Source: CAD feature listing. Evaluate the final solid. Frame: model axes, mm. Face numbers are marked on the shaded views. A direction names the side the tool comes from. Round coordinates to 2 decimals unless told otherwise and drop trailing zeros. Order: outer loops, then holes, each group sorted by start corner. A loop starts at its lowest first (then second) coordinate and runs counter-clockwise, first axis right, second up. Notation, with made-up numbers: M 86,77.25 L 142,77.25 A34 ccw 142,110.25 Z; hole C -36.75,15.5 d1. An arc over 180 degrees is marked long. Answer as CSV lines item,"result". Start each with the question number.
Item 1: Section query B-B on x = 51. Return the cut outline in (y, z).
Item 2: Section query C-C on z = -55. Return the cut outline in (x, y), plus the area to 3 significant figures.
Item 3: Section query D-D on y = 27. Return the cut outline in (x, z), plus the area to 3 significant figures.
Item 4: Set-up query: the marked faces 1 and 2. Return all of +Z, -Z, +X, -X, +Y, -Y with unobstructed straight access to the full face (end or side cutting, diameter ignored); none if empty.
Item 5: Section query A-A on y = 47. Return the cut outline in (x, z), plus the area to 3 significant figures.
Item 6: First-contact query: P1, Ø2, axis at y = 32, z = -28, coming from the +X side; P2, Ø12, axis at x = 28.5, z = -23, coming from the +Y side; P3, Ø1.5, axis at y = 7, z = 2.5, coming from the +X side. Flat tips, straight axial feed; report the tip coordinate or a pass-through.
Item 7: Line query: line 1 (Y direction, x = 24, z = -10); line 2 (X direction, y = 7, z = -67). Output: solid intervals per line, ascending. Write a range as [from, to].
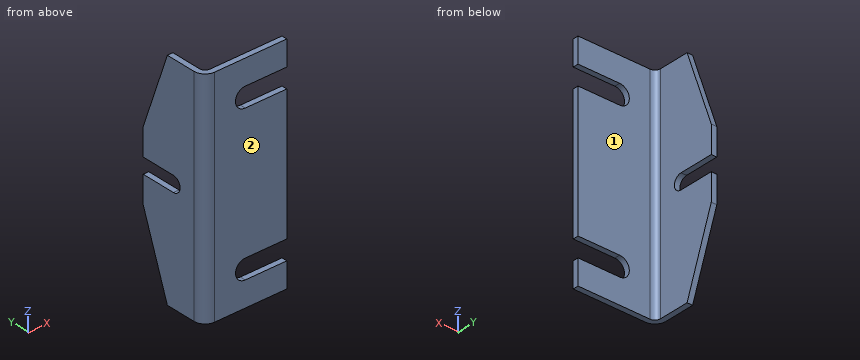
from build123d import *

# Parameters (mm, degrees)
BASE_FLANGE3_DEPTH = 80
CUT_EXTRUDE1_DEPTH = 110.708705215
CUT_EXTRUDE2_DEPTH = 111.072703247


# Sheet-metal steps are written as plain solids
with BuildPart() as part:
    # Sketch1 → Base-Flange3 (new, symmetric)
    with BuildSketch(Plane.XY):
        with BuildLine():
            Line((60, 0), (8, 0))
            ThreePointArc((8, 0), (2.343145751, 2.343145751), (0, 8))
            Line((0, 8), (0, 50))
            Line((0, 50), (4, 50))
            Line((4, 50), (4, 8))
            ThreePointArc((4, 8), (5.171572875, 5.171572875), (8, 4))
            Line((8, 4), (60, 4))
            Line((60, 4), (60, 0))
        make_face()
    extrude(amount=BASE_FLANGE3_DEPTH, both=True)

    # Sketch14 → Cut-Extrude1 (cut, through all)
    with BuildSketch(Plane(origin=(4, 0, 0), x_dir=(0, 0, -1), z_dir=(1, 0, 0))):
        Polygon((-80, 30), (-25, 50), (-80, 50), align=None)
        Polygon((80, 30), (25, 50), (80, 50), align=None)
        with BuildLine():
            Line((-5.5, 50), (-5.5, 25))
            ThreePointArc((-5.5, 25), (0, 19.5), (5.5, 25))
            Line((5.5, 25), (5.5, 50))
            Line((5.5, 50), (-5.5, 50))
        make_face()
    extrude(amount=-CUT_EXTRUDE1_DEPTH, mode=Mode.SUBTRACT)

    # Sketch16 → Cut-Extrude2 (cut, through all)
    with BuildSketch(Plane(origin=(0, 4, 0), x_dir=(1, 0, 0), z_dir=(0, 1, 0))):
        with BuildLine():
            Line((60, 62), (30, 62))
            ThreePointArc((30, 62), (23, 55), (30, 48))
            Line((30, 48), (60, 48))
            Line((60, 48), (60, 62))
        make_face()
        with BuildLine():
            Line((60, -48), (60, -62))
            Line((60, -62), (30, -62))
            ThreePointArc((30, -62), (23, -55), (30, -48))
            Line((30, -48), (60, -48))
        make_face()
    extrude(amount=-CUT_EXTRUDE2_DEPTH, mode=Mode.SUBTRACT)


solid = part.part
Results:
1,outline,"M 0,-80 L 4,-80 L 4,-62 L 0,-62 Z; M 0,-48 L 4,-48 L 4,48 L 0,48 Z; M 0,62 L 4,62 L 4,80 L 0,80 Z"
2,outline,"M 0,8 A8 ccw 8,0 L 23,0 L 23,4 L 8,4 A4 cw 4,8 L 4,39.09 L 0,39.09 Z"
2,area,"222 mm^2"
3,outline,"M 0,-80 L 4,-80 L 4,-5.5 L 0,-5.5 Z; M 0,5.5 L 4,5.5 L 4,80 L 0,80 Z"
3,area,"596 mm^2"
4,face 1,"+Z, -Z, +X, +Y"
4,face 2,"+Z, -Z, +X, -X, -Y"
5,outline,"M 0,-33.25 L 4,-33.25 L 4,-5.5 L 0,-5.5 Z; M 0,5.5 L 4,5.5 L 4,33.25 L 0,33.25 Z"
5,area,"222 mm^2"
6,P1,"x = 4"
6,P2,"y = 4"
6,P3,"x = 4.4"
7,line 1,"[0, 4]"
7,line 2,"[0.06, 4.13]"
